For this review, take the finished solid that the model builds, in its own axes (mm). Give positions to 0.01 mm unless a question says otherwise; leave off trailing zeros. Write each loop counter-clockwise with the first axis right and the second up, starting at its lowest first coordinate (ties: lowest second). Pieces come first, ordered by that corner, then holes.
1) We need section B-B on x = -6.35. Give the boundary of the cut face in (y, z) (1 decimal), and give its area (3 significant figures).
2) We need section C-C on y = 101. Give the boundary of the cut face in (x, z) (3 decimals).
3) We need section A-A on x = -54.61. Give the boundary of the cut face in (y, z) (1 decimal), and give its area (3 significant figures).
4) We need section D-D on z = -1.35. Give the number of separate pieces and of enclosed holes in the cut face, and give its area (3 significant figures).
5) Wall thickness on line 1 along Y through (x, z) = (-33, -0.5); line 2 along Y through (x, z) = (-37.5, -1.35); line 3 along X through (y, z) = (78, -1.9): over which ranges is each line inside the solid? List them lowest first.
6) For P1, Ø1, axis at y = 2.5, z = -1, coming from the -X side; P2, Ø1, axis at y = 58.5, z = -1.5, coming from the -X side; P3, Ø1.6, axis at x = -55, z = -1.5, coming from the -Y side, all flat-tipped, find the tip position at first contact; note any pin that passes through.
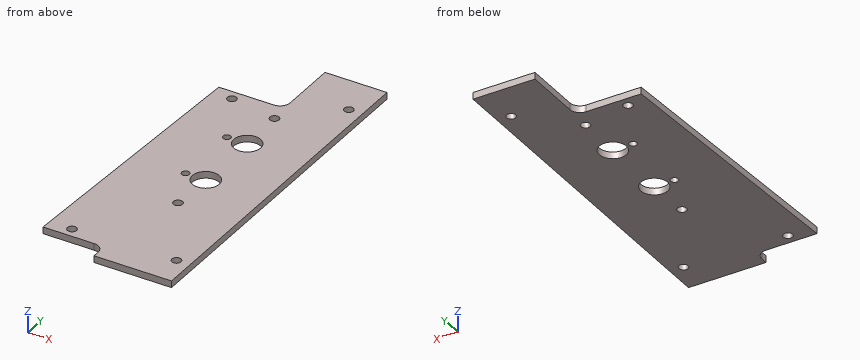
from build123d import *

# Parameters (mm, degrees)
BOSS_EXTRUDE1_DEPTH             = 3.175
F_9_64_0_14063_DIAMETER_HOLE1_D = 3.572002
F_1_2_0_5_DIAMETER_HOLE1_D      = 12.7
F_6_CLEARANCE_HOLE1_D           = 4.3053
F_6_CLEARANCE_HOLE2_D           = 4.3053
SKETCH13_W                      = 23.574867554
SKETCH13_H                      = 15.925568069
BOSS_EXTRUDE2_DEPTH             = 3.175


with BuildPart() as part:
    # Sketch1 → Boss-Extrude1 (new body)
    with BuildSketch(Plane.XY):
        with BuildLine():
            Line((-36.5125, 0), (0, 0))
            Line((0, 0), (0, 166.6875))
            Line((0, 166.6875), (-29.21, 166.6875))
            Line((-29.21, 166.6875), (-29.21, 139.7))
            ThreePointArc((-29.21, 139.7), (-30.604903955, 136.332403955), (-33.9725, 134.9375))
            Line((-33.9725, 134.9375), (-59.89066, 134.9375))
            Line((-59.89066, 134.9375), (-65.379450588, 7.9375))
            Line((-65.379450588, 7.9375), (-41.275, 7.9375))
            ThreePointArc((-41.275, 7.9375), (-37.907403955, 6.542596045), (-36.5125, 3.175))
            Line((-36.5125, 3.175), (-36.5125, 0))
        make_face()
    extrude(amount=-BOSS_EXTRUDE1_DEPTH)

    # 9/64 (0.14063) Diameter Hole1 (through all)
    with Locations(Plane.XY):
        with Locations((-18.415, 26.3525), (-37.465, 72.39), (-37.465, 104.394)):
            Hole(F_9_64_0_14063_DIAMETER_HOLE1_D / 2)

    # 1/2 (0.5) Diameter Hole1 (through all)
    with Locations(Plane.XY):
        with Locations((-27.94, 26.3525), (-27.94, 72.39), (-27.94, 104.394)):
            Hole(F_1_2_0_5_DIAMETER_HOLE1_D / 2)

    # #6 Clearance Hole1 (through all)
    with Locations(Plane.XY):
        with Locations((-28.448, 51.7525), (-28.448, 126.365)):
            Hole(F_6_CLEARANCE_HOLE1_D / 2)

    # #6 Clearance Hole2 (through all)
    with Locations(Plane.XY):
        with Locations((-50.8, 130.175), (-6.35, 147.6375), (-6.35, 14.2875), (-54.61, 12.7)):
            Hole(F_6_CLEARANCE_HOLE2_D / 2)

    # Sketch13 → Boss-Extrude2 (add, through all)
    with BuildSketch(Plane.XY):
        with Locations((-24.941412977, 26.424397309)):
            Rectangle(SKETCH13_W, SKETCH13_H)
    extrude(amount=-BOSS_EXTRUDE2_DEPTH)


solid = part.part
Results list:
1. outline: (0, -3.2) - (12.1, -3.2) - (12.1, 0) - (0, 0) - close; (16.4, -3.2) - (145.5, -3.2) - (145.5, 0) - (16.4, 0) - close; (149.8, -3.2) - (166.7, -3.2) - (166.7, 0) - (149.8, 0) - close
1. area: 502 mm2
2. outline: (-61.357, -3.175) - (-33.307, -3.175) - (-33.307, 0) - (-61.357, 0) - close; (-22.573, -3.175) - (0, -3.175) - (0, 0) - (-22.573, 0) - close
3. outline: (7.9, -3.2) - (10.5, -3.2) - (10.5, 0) - (7.9, 0) - close; (14.9, -3.2) - (134.9, -3.2) - (134.9, 0) - (14.9, 0) - close
3. area: 390 mm2
4. separate pieces: 1
4. enclosed holes: 10
4. area: 8,820 mm2
5. line 1: y = 0 to 68.55, 76.23 to 100.56, 108.23 to 135.04
5. line 2: y = 6.08 to 70.6, 74.18 to 102.61, 106.18 to 134.94
5. line 3: x = -62.35 to -30.91, -24.97 to 0
6. P1: stops at x = -36.51
6. P2: stops at x = -63.22
6. P3: stops at y = 7.94
